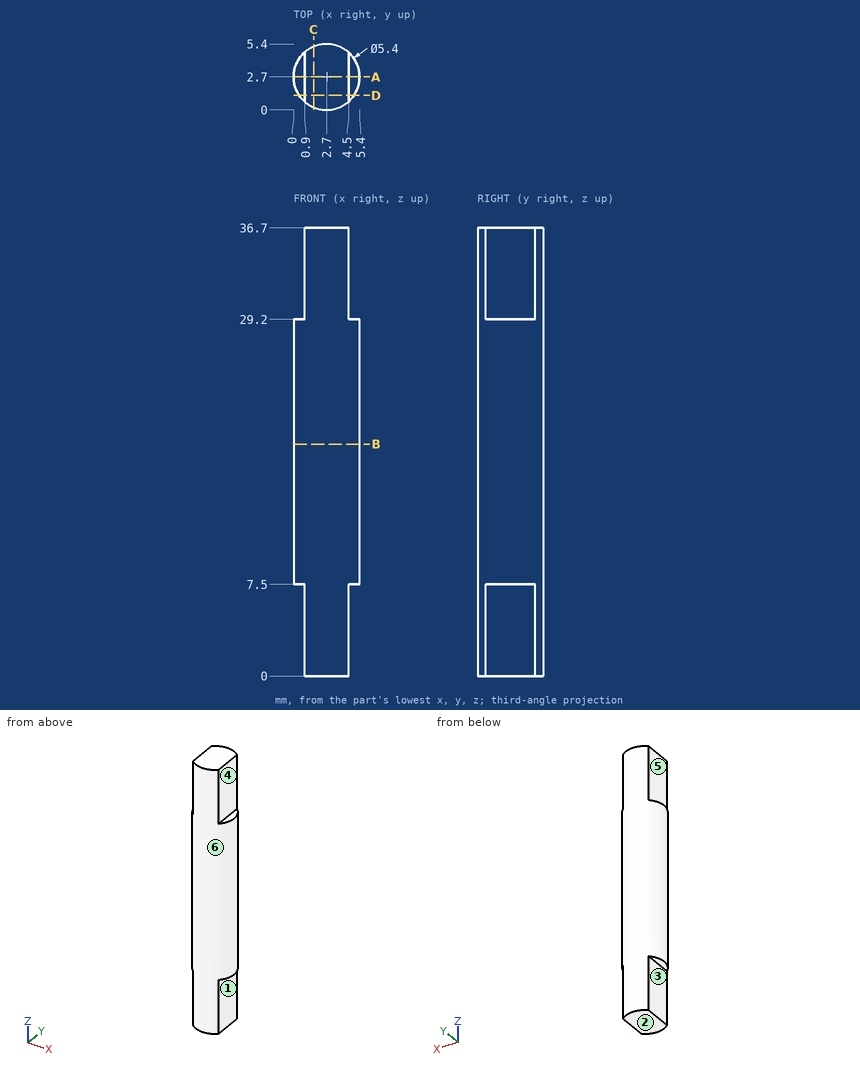
The drawing under review shows one solid part. Ordinate dimensions are in mm from its lowest x, y, z. A direction names the side the tool comes from. Coordinates: 2 decimals unless noted, no trailing zeros. Order: outer loops, then holes, each group sorted by start corner. A loop starts at its lowest first (then second) coordinate and runs counter-clockwise, first axis right, second up. Notation, with made-up numbers: (10, -15.5) -> (33, -15.5) arc R23 cw to (33, 16.5) -> close; hole circle Ø8 at (14, 40). An arc over 180 degrees is marked (long way). Return JSON: item names as keys, results as strings.
1. For pin 1 Ø3 at (y, z) = (2, 31.5) entering from +X; pin 2 Ø0.5 at (x, y) = (0.5, 1.5) entering from -Z; pin 3 Ø1 at (x, z) = (5, 15.5) entering from -Y, all flat-tipped, find the tip position at first contact; note any pin that passes through.
Answer block:
{"pin 1": "x = 4.5", "pin 2": "z = 7.5", "pin 3": "y = 0.69"}
2. We need section B-B on z = 19. Write out the cut boundary in (x, y).
Answer block:
{"outline": "circle Ø5.4 at (2.7, 2.7)"}
3. Machinability: for the marked faces 1, 2, 3 and 4, which of the approach directions +Z, -Z, +X, -X, +Y, -Y give a long, thin tool a straight path to every point of the face, cutting with its end or side? Answer none if there is none.
Answer block:
{"face 1": "-Z, +X, +Y, -Y", "face 2": "-Z, +X, -X, +Y, -Y", "face 3": "-Z, -X, +Y, -Y", "face 4": "+Z, +X, +Y, -Y"}
4. The part is to be moulded in two halves that separate along Y. For the marked faces 5 and 6, say which applies: +Y half, -Y half, draft (parallel to the pull), parting line (faces both ways), or undercut.
Answer block:
{"face 5": "draft", "face 6": "parting line"}
5. We need section C-C on x = 1.65. Write out the cut boundary in (y, z).
Answer block:
{"outline": "(0.21, 0) -> (5.19, 0) -> (5.19, 36.7) -> (0.21, 36.7) -> close"}
6. For line 1 (Z direction, x = 0.75, y = 1.2); line 2 (X direction, y = 3.9, z = 3.5); line 3 (Y direction, x = 2.6, z = 34), list the stretches that pass through material, from the lowest coordinate up. Write a range as from..to.
Answer block:
{"line 1": "7.5..29.2", "line 2": "0.9..4.5", "line 3": "0..5.4"}
7. We need section A-A on y = 2.7. Write out the cut boundary in (x, z).
Answer block:
{"outline": "(0, 7.5) -> (0.9, 7.5) -> (0.9, 0) -> (4.5, 0) -> (4.5, 7.5) -> (5.4, 7.5) -> (5.4, 29.2) -> (4.5, 29.2) -> (4.5, 36.7) -> (0.9, 36.7) -> (0.9, 29.2) -> (0, 29.2) -> close"}
8. We need section D-D on y = 1.2. Write out the cut boundary in (x, z) (3 decimals).
Answer block:
{"outline": "(0.455, 7.5) -> (0.9, 7.5) -> (0.9, 0) -> (4.5, 0) -> (4.5, 7.5) -> (4.945, 7.5) -> (4.945, 29.2) -> (4.5, 29.2) -> (4.5, 36.7) -> (0.9, 36.7) -> (0.9, 29.2) -> (0.455, 29.2) -> close"}
